Source: CAD feature listing. Evaluate the final solid. Frame: model axes, mm. A direction names the side the tool comes from. Give positions to 0.01 mm unless a question says otherwise; leave off trailing zeros. Write each loop counter-clockwise with the first axis right and the second up, starting at its lowest first coordinate (ties: lowest second). Pieces come first, ordered by that corner, then holes. Notation, with made-up numbers: M -16.5,49 L 16.5,49 A14 ccw 16.5,53 Z; hole C 4,-29.5 d8. An arc over 180 degrees is marked long. Return JSON: item names as keys, results as strings.
Autodesk Inventor part; units mm, degrees
ref_plane "YZ Plane" through (0, 0, 0) normal (1, 0, 0) x (0, 1, 0)
ref_plane "XZ Plane" through (0, 0, 0) normal (0, 1, 0) x (-1, 0, 0)
ref_plane "XY Plane" through (0, 0, 0) normal (0, 0, 1) x (1, 0, 0)
sketch "Sketch1" plane through (0, 0, 0) normal (0, 0, 1) x (1, 0, 0)
  line L0 (-27.5, 79) -> (27.5, 79)
  line L1 (27.5, 79) -> (27.5, -79)
  line L2 (27.5, -79) -> (-27.5, -79)
  line L3 (-27.5, -79) -> (-27.5, 79)
  line L4 (-20, 71.5) -> (20, 71.5)
  line L5 (20, 71.5) -> (20, -71.5)
  line L6 (20, -71.5) -> (-20, -71.5)
  line L7 (-20, -71.5) -> (-20, 71.5)
  point P0 (0, 0)
  point P1 (0, -79)
  dimension "d0" = 55
  dimension "d1" = 158
  dimension "d2" = 79
  dimension "d3" = 27.5
  dimension "d4" = 143
  dimension "d5" = 40
  dimension "d6" = 20
  dimension "d7" = 71.5
extrude "Extrusion1" add sketch "Sketch1" along normal mid plane 3
sketch "Sketch2" plane through (-27.5, 79, -1.5) normal (0, 1, 0) x (1, 0, 0)
  circle A0 centre (27.5, -1.5) radius 28
  point P0 (27.5, -1.5)
  dimension "d10" = 56
extrude "Extrusion2" add sketch "Sketch2" against normal blind 8
sketch "Sketch3" plane through (0, 0, 1.5) normal (0, 0, 1) x (1, 0, 0)
  line L0 (-25, 71) -> (25, 71)
  line L1 (25, 71) -> (25, -9)
  line L2 (25, -9) -> (-25, -9)
  line L3 (-25, -9) -> (-25, 71)
  circle A0 centre (-22, -6) radius 1.5
  circle A1 centre (-22, 68) radius 1.5
  circle A2 centre (22, -6) radius 1.5
  circle A3 centre (22, 68) radius 1.5
  line L4 (-28, 71) -> (28, 71)
  point P0 (0, 0)
  dimension "d13" = 80
  dimension "d14" = 50
  dimension "d15" = 25
  dimension "d16" = 3
  dimension "d18" = 3
  dimension "d19" = 3
  dimension "d20" = 3
  dimension "d21" = 44
  dimension "d22" = 44
  dimension "d23" = 22
  dimension "d24" = 22
  dimension "d25" = 74
  dimension "d27" = 74
  dimension "d77" = 0
  dimension "d78" = 3
  dimension "d79" = 3
extrude "Extrusion3" cut sketch "Sketch3" against normal blind 6 contours A0 | A1 | A2 | A3
sketch "Sketch4" plane through (-27.5, -79, 1.5) normal (0, -1, 0) x (1, 0, 0)
  circle A0 centre (27.5, -1.5) radius 28
  point P0 (27.5, -1.5)
extrude "Extrusion4" add sketch "Sketch4" along normal blind 8
sketch "Sketch5" plane through (0, 0, 0) normal (1, 0, 0) x (0, 1, 0)
  circle A0 centre (-81.5, 0) radius 1.5
  line L0 (-79, 28) -> (-79, -28)
  point P0 (0, 0)
  dimension "d33" = 3
  dimension "d34" = 2.5
extrude "Extrusion5" cut sketch "Sketch5" along normal through all both and the other way through all
thread "Thread1"
sketch "Sketch6" plane through (0, -87, 0) normal (0, -1, 0) x (1, 0, 0)
  circle A0 centre (0, 0) radius 25
  circle A1 centre (0, 0) radius 22.5
  point P0 (0, 0)
  dimension "d39" = 50
  dimension "d40" = 45
extrude "Extrusion6" add sketch "Sketch6" along normal blind 5
thread "Thread2"
sketch "Sketch7" plane through (0, -79, 0) normal (0, 1, 0) x (1, 0, 0)
  circle A0 centre (0, 0) radius 22.5
  line L0 (14.7394, 17) -> (-15.2606, 17)
  line L1 (-15.2606, 17) -> (-15.2606, 8)
  line L2 (-15.2606, 8) -> (14.7394, 8)
  line L3 (14.7394, 8) -> (14.7394, 17)
  line L4 (14.7394, -7.5337) -> (-15.2606, -7.5337)
  line L5 (-15.2606, -7.5337) -> (-15.2606, -16.5337)
  line L6 (-15.2606, -16.5337) -> (14.7394, -16.5337)
  line L7 (14.7394, -16.5337) -> (14.7394, -7.5337)
  point P0 (0, 0)
  point P1 (-14.7394, 17)
  point P2 (-15.2606, 16.5337)
  dimension "d45" = 9
  dimension "d46" = 9
  dimension "d47" = 30
  dimension "d48" = 8
extrude "Extrusion7" cut sketch "Sketch7" against normal blind 10 contours L5 L4 L7 L6 | L3 L2 L1 A0 L0
sketch "Sketch8" plane through (0, 79, 0) normal (0, 1, 0) x (1, 0, 0)
  circle A0 centre (0, -17) radius 1.5
  circle A1 centre (-17, 0) radius 1.5
  circle A2 centre (0, 17) radius 1.5
  circle A3 centre (17, 0) radius 1.5
  point P0 (0, 0)
  dimension "d51" = 3
  dimension "d52" = 3
  dimension "d53" = 3
  dimension "d54" = 3
  dimension "d55" = 34
  dimension "d56" = 34
  dimension "d57" = 17
  dimension "d58" = 17
extrude "Extrusion8" cut sketch "Sketch8" against normal blind 10
sketch "Sketch10" plane through (0, 79, 0) normal (0, 1, 0) x (1, 0, 0)
  circle A0 centre (0, 0) radius 28
  circle A1 centre (0, 0) radius 26.5
  point P0 (0, 0)
  dimension "d80" = 53
  dimension "d81" = 56
extrude "Extrusion10" add sketch "Sketch10" along normal blind 5
thread "Thread3"
sketch "Sketch11" plane through (0, 79, 0) normal (0, 1, 0) x (1, 0, 0)
  circle A0 centre (0, 0) radius 25
  circle A1 centre (0, 25) radius 1.5
  point P0 (0, 0)
  dimension "d86" = 3
extrude "Extrusion11" cut sketch "Sketch11" against normal up to surface (8 mm away) contours A1 A0 | A0 A1 picked at (-0.0591, 24.5002) picked at (0.0534, 25.4938)
pattern_circular "Circular Pattern1" count 10 over 360 about axis through (0, 79, 0) along (0, -1, 0) of "Extrusion11"
sketch "Sketch12" plane through (0, 0, -1.5) normal (0, 0, -1) x (-1, 0, 0)
  circle A0 centre (-22, -89.4052) radius 1.5
  point P0 (0, 0)
  dimension "d93" = 3
  dimension "d94" = 22
extrude "Extrusion12" cut sketch "Sketch12" against normal blind 10
pattern_linear "Rectangular Pattern1" count 2 spacing 100 along (0, -1, 0) of "Extrusion3"
sketch "Sketch13" plane through (0, 79, -25) normal (0, 1, 0) x (1, 0, 0)
  circle A0 centre (9, -34) radius 5
  line L0 (14.7394, -17) -> (-15.2606, -17)
  circle A1 centre (9, -16) radius 5
  circle A2 centre (-9, -16) radius 5
  circle A3 centre (-9, -34) radius 5
  point P0 (0, -25)
  dimension "d100" = 10
  dimension "d101" = 10
  dimension "d104" = 18
  dimension "d108" = 9
  dimension "d109" = 9
  dimension "d110" = 9
  dimension "d111" = 10
  dimension "d112" = 10
  dimension "d113" = 9
  dimension "d114" = 9
  dimension "d115" = 9
  dimension "d116" = 9
extrude "Extrusion13" cut sketch "Sketch13" against normal up to surface (8 mm away)
sketch "Sketch14" plane through (-20, -71.5, 1.5) normal (0, 1, 0) x (1, 0, 0)
  arc A0 (4.7394, 18.0337) -> (4.7394, -15.0337) centre (20, 1.5) ccw
  line L0 (-7.5, 0) -> (47.5, 0)
  line L1 (-2.4455, 3.065) -> (42.5703, 3.065)
  line L2 (42.5703, 3.065) -> (42.5703, 0)
  line L3 (42.5703, 0) -> (-2.4455, 0)
  line L4 (-2.4455, 0) -> (-2.4455, 3.065)
  point P0 (20, 1.5)
  point P1 (-2.4455, 0)
extrude "Extrusion14" add sketch "Sketch14" along normal up to surface (142.5 mm away) contours L1 L2 L0 L4
ref_plane "Work Plane1" through (0, 0, 61.5) normal (0, 0, 1) x (1, 0, 0)
sketch "Sketch15" plane through (0, 0, 61.5) normal (0, 0, 1) x (1, 0, 0)
  line L0 (-22.4455, 66.5677) -> (-22.4455, -4.5677)
  line L1 (-22.4455, 66.5) -> (20.5545, 66.5)
  line L2 (20.5545, 66.5) -> (20.5545, -66.5)
  line L3 (20.5545, -66.5) -> (-22.4455, -66.5)
  line L4 (-22.4455, -66.5) -> (-22.4455, 66.5)
  line L5 (-22.4455, 56.5) -> (20.5545, 56.5)
  line L6 (-22.4455, 46.5) -> (20.5545, 46.5)
  line L7 (-22.4455, 36.5) -> (20.5545, 36.5)
  line L8 (-22.4455, 26.5) -> (20.5545, 26.5)
  line L9 (-22.4455, 16.5) -> (20.5545, 16.5)
  line L10 (-22.4455, 6.5) -> (20.5545, 6.5)
  line L11 (-22.4455, -3.5) -> (20.5545, -3.5)
  line L12 (-22.4455, -13.5) -> (20.5545, -13.5)
  line L13 (-22.4455, -23.5) -> (20.5545, -23.5)
  line L14 (-22.4455, -33.5) -> (20.5545, -33.5)
  line L15 (-22.4455, -43.5) -> (20.5545, -43.5)
  line L16 (-22.4455, -53.5) -> (20.5545, -53.5)
  line L17 (-22.4455, -63.5) -> (20.5545, -63.5)
  line L18 (15.5545, 66.5) -> (15.5545, -66.5)
  line L19 (10.5545, 66.5) -> (10.5545, -66.5)
  line L20 (5.5545, 66.5) -> (5.5545, -66.5)
  line L21 (0.5545, 66.5) -> (0.5545, -66.5)
  line L22 (-4.4455, 66.5) -> (-4.4455, -66.5)
  line L23 (-9.4455, 66.5) -> (-9.4455, -66.5)
  line L24 (-14.4455, 66.5) -> (-14.4455, -66.5)
  line L25 (-19.4455, 66.5) -> (-19.4455, -66.5)
  line L26 (-24.4455, 66.5) -> (-24.4455, -66.5)
  point P0 (0, 0)
  point P1 (15.5545, -43.5)
  point P2 (15.5545, -53.5)
  point P3 (5.5545, -43.5)
  point P4 (5.5545, -53.5)
  point P5 (10.5545, -53.5)
  point P6 (10.5545, -43.5)
  point P7 (-4.4455, -43.5)
  point P8 (-4.4455, -53.5)
  point P9 (0.5545, -53.5)
  point P10 (0.5545, -43.5)
  point P11 (-14.4455, -43.5)
  point P12 (-14.4455, -53.5)
  point P13 (-9.4455, -53.5)
  point P14 (-9.4455, -43.5)
  point P15 (-19.4455, -53.5)
  point P16 (-19.4455, -43.5)
  point P17 (10.5545, -23.5)
  point P18 (10.5545, -33.5)
  point P19 (15.5545, -33.5)
  point P20 (15.5545, -23.5)
  point P21 (0.5545, -23.5)
  point P22 (0.5545, -33.5)
  point P23 (5.5545, -33.5)
  point P24 (5.5545, -23.5)
  point P25 (-9.4455, -23.5)
  point P26 (-9.4455, -33.5)
  point P27 (-4.4455, -33.5)
  point P28 (-4.4455, -23.5)
  point P29 (-19.4455, -23.5)
  point P30 (-19.4455, -33.5)
  point P31 (-14.4455, -33.5)
  point P32 (-14.4455, -23.5)
  point P33 (15.5545, -3.5)
  point P34 (15.5545, -13.5)
  point P35 (5.5545, -3.5)
  point P36 (5.5545, -13.5)
  point P37 (10.5545, -13.5)
  point P38 (10.5545, -3.5)
  point P39 (-4.4455, -3.5)
  point P40 (-4.4455, -13.5)
  point P41 (0.5545, -13.5)
  point P42 (0.5545, -3.5)
  point P43 (-14.4455, -3.5)
  point P44 (-14.4455, -13.5)
  point P45 (-9.4455, -13.5)
  point P46 (-9.4455, -3.5)
  point P47 (-19.4455, -13.5)
  point P48 (-19.4455, -3.5)
  point P49 (-22.4455, -4.5677)
  point P50 (15.5545, 16.5)
  point P51 (15.5545, 6.5)
  point P52 (5.5545, 16.5)
  point P53 (5.5545, 6.5)
  point P54 (10.5545, 6.5)
  point P55 (10.5545, 16.5)
  point P56 (-4.4455, 16.5)
  point P57 (-4.4455, 6.5)
  point P58 (0.5545, 6.5)
  point P59 (0.5545, 16.5)
  point P60 (-14.4455, 16.5)
  point P61 (-14.4455, 6.5)
  point P62 (-9.4455, 6.5)
  point P63 (-9.4455, 16.5)
  point P64 (-19.4455, 6.5)
  point P65 (-19.4455, 16.5)
  point P66 (-19.4455, 36.5)
  point P67 (-19.4455, 26.5)
  point P68 (-14.4455, 26.5)
  point P69 (-14.4455, 36.5)
  point P70 (-19.4455, 56.5)
  point P71 (-19.4455, 46.5)
  point P72 (-14.4455, 46.5)
  point P73 (-14.4455, 56.5)
  point P74 (-9.4455, 56.5)
  point P75 (-9.4455, 46.5)
  point P76 (-4.4455, 46.5)
  point P77 (-4.4455, 56.5)
  point P78 (-9.4455, 36.5)
  point P79 (-9.4455, 26.5)
  point P80 (-4.4455, 26.5)
  point P81 (-4.4455, 36.5)
  point P82 (10.5545, 36.5)
  point P83 (10.5545, 26.5)
  point P84 (15.5545, 26.5)
  point P85 (15.5545, 36.5)
  point P86 (10.5545, 56.5)
  point P87 (10.5545, 46.5)
  point P88 (15.5545, 46.5)
  point P89 (15.5545, 56.5)
  point P90 (0.5545, 56.5)
  point P91 (0.5545, 46.5)
  point P92 (5.5545, 46.5)
  point P93 (5.5545, 56.5)
  point P94 (0.5545, 36.5)
  point P95 (0.5545, 26.5)
  point P96 (5.5545, 26.5)
  point P97 (5.5545, 36.5)
  dimension "d122" = 43
  dimension "d123" = 133
  dimension "d124" = 66.5
  dimension "d127" = 10
  dimension "d134" = 5
extrude "Extrusion15" cut sketch "Sketch15" against normal up to surface (63.065 mm away) contours L5 L24 L6 L25 | L7 L24 L8 L25 | L5 L22 L6 L23 | L9 L25 L10 L0 | L7 L22 L8 L23 | L5 L20 L6 L21 | L11 L25 L12 L4 L0 | L9 L23 L10 L24 | L7 L20 L8 L21 | L5 L18 L6 L19 | L11 L23 L12 L24 | L9 L21 L10 L22 | L13 L24 L14 L25 | L7 L18 L8 L19 | L11 L21 L12 L22 | L9 L19 L10 L20 | L15 L25 L16 L4 | L13 L22 L14 L23 | L11 L19 L12 L20 | L15 L23 L16 L24 | L9 L2 L10 L18 | L13 L20 L14 L21 | L11 L2 L12 L18 | L15 L21 L16 L22 | L13 L18 L14 L19 | L15 L19 L16 L20 | L15 L2 L16 L18
ref_plane "Work Plane2" through (0, -79, 0) normal (0, 1, 0) x (1, 0, 0)
split "Split1" plane through (0, -79, 0) removes the side toward (0, 1, 0)
sketch "Sketch16" plane through (0, -79, 0) normal (0, 1, 0) x (1, 0, 0)
  line L0 (-28, 1.5) -> (28, 1.5)
  line L1 (28, 1.5) -> (28, -1.5)
  line L2 (28, -1.5) -> (-28, -1.5)
  line L3 (-28, -1.5) -> (-28, 1.5)
  point P0 (0, 0)
  dimension "d142" = 3
  dimension "d143" = 1.5
  dimension "d144" = 56
  dimension "d145" = 28
extrude "Extrusion16" cut sketch "Sketch16" against normal blind 5
properties part number "case v0 bottom"
1) Line query: line 1 (Z direction, x = 0, y = -84.75); line 2 (Z direction, x = 0, y = -81.25); line 3 (Z direction, x = -0.5, y = -89) (3 decimals). Output: solid intervals per line, ascending. Write a range as [from, to].
Numbers:
{"line 1": "z = [-28, -17], [-8, 7.53], [16.53, 28]", "line 2": "z = [-28, -17], [-8, -1.5], [1.5, 7.53], [16.53, 28]", "line 3": "z = [-24.995, -22.494], [22.494, 24.995]"}
2) Cut plane C-C, the plane z = -14. Return the cut outline in (x, y), then the cut area to 3 significant figures.
Numbers:
{"outline": "M -24.25,-87 L -20.71,-87 L -20.71,-92 L -17.61,-92 L -17.61,-87 L -15.26,-87 L -15.26,-79 L -24.25,-79 Z; M 14.74,-87 L 17.61,-87 L 17.61,-92 L 20.71,-92 L 20.71,-87 L 24.25,-87 L 24.25,-79 L 14.74,-79 Z", "area": "179 mm²"}
3) Cut plane D-D, the plane x = -18. Return the cut outline in (y, z), then the cut area to 3 significant figures.
Numbers:
{"outline": "M -92,-17.35 L -87,-17.35 L -87,-21.45 L -79,-21.45 L -79,-1.5 L -84,-1.5 L -84,1.5 L -79,1.5 L -79,21.45 L -87,21.45 L -87,17.35 L -92,17.35 L -92,13.5 L -87,13.5 L -87,-13.5 L -92,-13.5 Z", "area": "367 mm²"}
4) Contact query for flat-ended pins moving along their axis: pin 1 Ø17 at (x, z) = (1, 5) entering from -Y; pin 2 Ø6.5 at (y, z) = (-84.5, 13.5) entering from +X; pin 3 Ø3 at (x, z) = (-8, -14) entering from +Y; pin 4 Ø6.5 at (y, z) = (-82.5, -12) entering from +X. Output: stop coordinate, or through.
Numbers:
{"pin 1": "stops at y = -87", "pin 2": "stops at x = 26.06", "pin 3": "passes through", "pin 4": "stops at x = 26.6"}
5) Set-up query: faces 4 (the face through (-11, -87, 23)), 5 (the face through (22, -89, 8.5)), 6 (the face through (-22.34, -92, 3.82)), 7 (the face through (0, -83, 16.534)), 8 (the face through (0, -84, 0)). Return all of +Z, -Z, +X, -X, +Y, -Y with unobstructed straight access to the full face (end or side cutting, diameter ignored); none if empty.
Numbers:
{"face 4": "-Y", "face 5": "none", "face 6": "+Z, -Z, +X, -X, -Y", "face 7": "+Y, -Y", "face 8": "+X, -X, +Y"}
6) Cut plane A-A, the plane y = -82. Return the cut outline in (x, z), then the cut area to 3 significant figures.
Numbers:
{"outline": "M -27.96,-1.5 A28 ccw 27.96,-1.5 Z; M -27.96,1.5 L 27.96,1.5 A28 ccw Z; hole M -15.26,-16.53 A22.5 ccw -14.74,-17 L 14.74,-17 L 14.74,-8 L -15.26,-8 Z; hole M -15.26,7.53 L 14.74,7.53 L 14.74,16.53 L -15.26,16.53 Z", "area": "1,760 mm²"}
7) Cut plane B-B, the plane x = 0. Return the cut outline in (y, z).
Numbers:
{"outline": "M -92,-25 L -87,-25 L -87,-28 L -79,-28 L -79,-17 L -87,-17 L -87,-22.5 L -92,-22.5 Z; M -92,22.5 L -87,22.5 L -87,16.53 L -79,16.53 L -79,28 L -87,28 L -87,25 L -92,25 Z; M -87,-8 L -79,-8 L -79,-1.5 L -84,-1.5 L -84,1.5 L -79,1.5 L -79,7.53 L -87,7.53 Z"}
8) Draft query along X for faces 1 (the face through (25.865, -82.944, 10.724)), 2 (the face through (0, -87, 3)), 3 (the face through (0, -81, -1.5)). Return one class per face: released by +X, released by -X, zero draft, split by the parting line, or undercut.
Numbers:
{"face 1": "split by the parting line", "face 2": "undercut", "face 3": "zero draft"}
